The drawing under review shows one solid part. Ordinate dimensions are in mm from its lowest x, y, z. Coordinates: 2 decimals unless noted, no trailing zeros. Write each loop counter-clockwise with the first axis right and the second up, starting at its lowest first coordinate (ties: lowest second). Pieces come first, ordered by that corner, then holes.
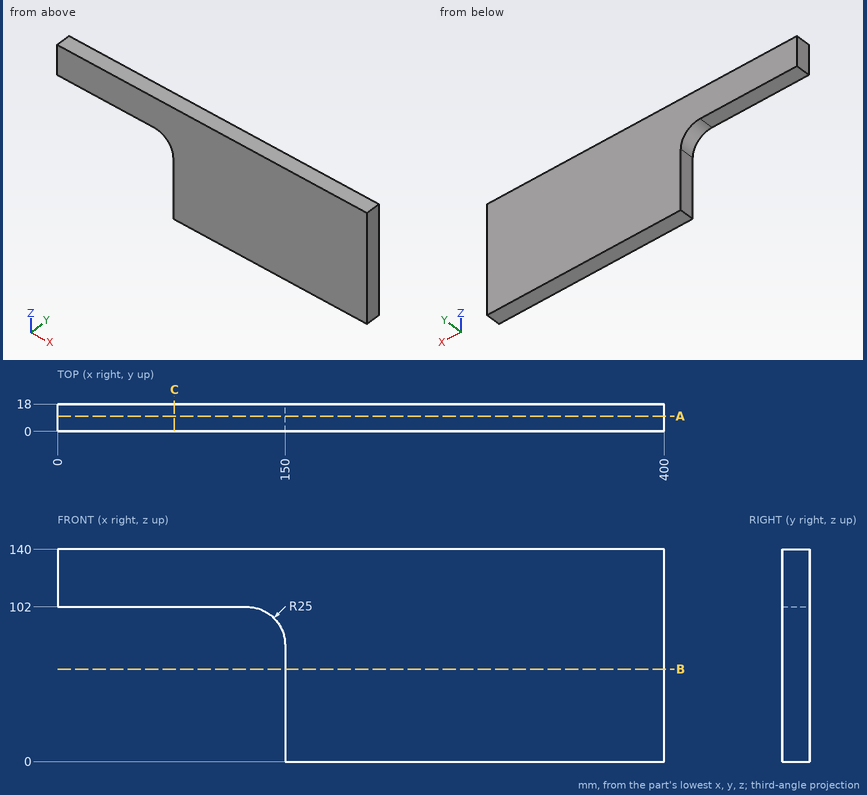
Q1. Add section B-B (z = 61). State the section outline as (x, y) points.
Ans:
outline: (150, 0) - (400, 0) - (400, 18) - (150, 18) - close
Q2. For probe 1 along X at (y, z) = (1, 11.5); probe 2 along Z at (x, y) = (26, 7); probe 3 along X at (y, z) = (1.5, 81), list the stretches that pass through material, from the lowest coordinate up.
Ans:
probe 1: x = 150 to 400
probe 2: z = 102 to 140
probe 3: x = 149.68 to 400
Q3. Add section C-C (x = 77). State the section outline as (y, z) points, then the cut area to 3 significant figures.
Ans:
outline: (0, 102) - (18, 102) - (18, 140) - (0, 140) - close
area: 684 mm2
Q4. Add section A-A (y = 10). State the section outline as (x, z) points, then the cut area to 3 significant figures.
Ans:
outline: (0, 102) - (125, 102) arc R25 cw to (150, 77) - (150, 0) - (400, 0) - (400, 140) - (0, 140) - close
area: 40,800 mm2
